Autodesk Inventor part; units mm, degrees
ref_plane "YZ Plane" through (0, 0, 0) normal (1, 0, 0) x (0, 1, 0)
ref_plane "XZ Plane" through (0, 0, 0) normal (0, 1, 0) x (-1, 0, 0)
ref_plane "XY Plane" through (0, 0, 0) normal (0, 0, 1) x (1, 0, 0)
sketch "Sketch1" plane through (0, 0, 0) normal (0, 0, 1) x (1, 0, 0)
  line L0 (-750, 48.2006) -> (750, 48.2006)
  line L1 (750, 48.2006) -> (750, 0)
  line L2 (750, 0) -> (-750, 0)
  line L3 (-750, 0) -> (-750, 48.2006)
  point P0 (0, 0)
  point P1 (0, 0)
  dimension "d0" = 1500
  dimension "d1" = 48.2006
extrude "Plate1" add sketch "Sketch1" along normal blind 3
sketch "Sketch2" plane through (750, 3, 0) normal (0, -1, 0) x (1, 0, 0)
  line L0 (-1500, 0) -> (0, 0)
  line L1 (0, 0) -> (0, 30)
  line L2 (0, 30) -> (-1500, 30)
  line L3 (-1500, 30) -> (-1500, 0)
edge flange "Flange1" height 30 angle 90 thickness 3 bend radius 3 thickness toward (0, -1, 0) relief tear relief width 3 relief depth 1.5 edges at (0, 0, 3) wall of the first edge with corners at (-750, 3, 0) (750, 3, 0) (750, 3, 30) (-750, 3, 30)
bend "Bend1"
corner "Corner1"
sketch "Sketch5" plane through (0, 0, 0) normal (0, 0, -1) x (-1, 0, 0)
  line L0 (750, 48.2006) -> (-750, 48.2006)
  line L1 (500, 48.2006) -> (500, 31)
  line L2 (500, 31) -> (503, 31)
  line L3 (503, 31) -> (503, 48.2006)
  line L4 (750, 0) -> (-750, 0)
  point P0 (0, 0)
  dimension "d18" = 3
  dimension "d19" = 247
  dimension "d20" = 31
extrude "Extrusion1" cut sketch "Sketch5" against normal through all
pattern_linear "Rectangular Pattern1" count 3 spacing 500 along (1, 0, 0) of "Extrusion1"
sketch "Sketch6" plane through (0, 0, 0) normal (0, 0, -1) x (-1, 0, 0)
  line L0 (-750, 48.2006) -> (-750, 6)
  circle A0 centre (-750, 48.2006) radius 15
  line L1 (-750, 48.2006) -> (-500, 48.2006)
  point P0 (0, 0)
  point P1 (-735, 48.2006)
  point P2 (-750, 33.2006)
  dimension "d24" = 30
extrude "Extrusion2" cut sketch "Sketch6" against normal through all contours L1 A0 L0 picked at (-740.1254, 47.088)
mirror "Mirror1" about plane through (0, 0, 0) normal (1, 0, 0) of "Extrusion2"
equation "\"d1\" = Стрингер_4"
equation "\"d18\" = Thickness"
equation "\"d2\" = Thickness"
equation "\"d3\" = BendReliefWidth"
equation "\"d4\" = BendReliefDepth"
equation "\"d5\" = MinimumRemnant"
equation "\"d6\" = TransitionRadius"
equation "\"d9\" = BendRadius"
equation "\"d10\" = CornerReliefSize"
equation "\"d11\" = GapSize"
equation "\"d12\" = JacobiRadiusSize"
equation "\"BendRadius\" = Thickness"
equation "\"BendReliefWidth\" = Thickness"
equation "\"BendReliefDepth\" = 0.5 * Thickness"
equation "\"CornerReliefSize\" = 4 * Thickness"
equation "\"MinimumRemnant\" = 2 * Thickness"
equation "\"TransitionRadius\" = BendRadius"
equation "\"JacobiRadiusSize\" = BendRadius"
equation "\"GapSize\" = Thickness"
properties part number "МОО 054 стрингер борт 41"
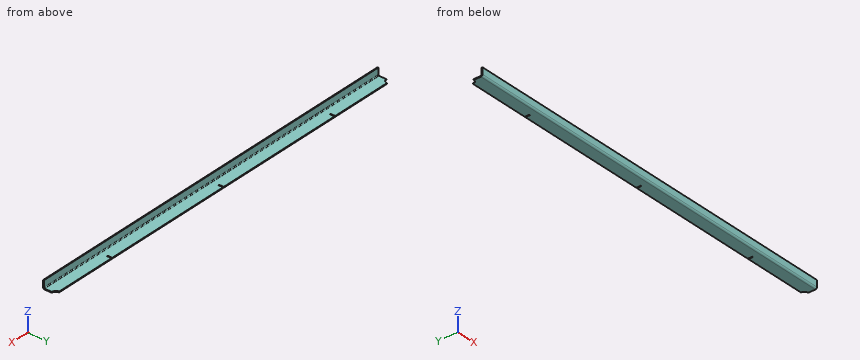
Input: part model. Units: mm. Frame: model coordinates. Give positions to 0.01 mm unless a question says otherwise; leave off trailing zeros. Order: outer loops, then holes, each group sorted by start corner. A loop starts at its lowest first (then second) coordinate and runs counter-clockwise, first axis right, second up. Notation, with made-up numbers: M -18.5,16.5 L 16.5,16.5 A29 ccw 16.5,41.5 Z; hole C -38.5,16.25 d7. An arc over 180 degrees is marked long. Return JSON: item names as keys, results as strings.
1) Line query: L1, parallel to Y at x = 185, z = 16.75; L2, parallel to Z at x = 522.5, y = 5. Output: solid intervals per line, ascending. Write a range as [from, to].
Taken from the geometry:
{"L1": "y = [0, 3]", "L2": "z = [0.08, 3.17]"}
2) Contact query for flat-ended pins moving along their axis: pin 1 (2.5 mm diameter, centred on y = 44, z = 1.5, fed in from -X); pin 2 (1.5 mm diameter, centred on x = -501, z = 1, fed in from +Y); pin 3 (1.5 mm diameter, centred on x = 46.5, z = 25, fed in from -Y); pin 4 (0.9 mm diameter, centred on y = 40.5, z = 2, fed in from -X). Output: stop coordinate, or through.
Taken from the geometry:
{"pin 1": "stops at x = -736.03", "pin 2": "stops at y = 31", "pin 3": "stops at y = 0", "pin 4": "stops at x = -737.41"}
3) Section query B-B on z = 12. Output: boundary loops of the cut face in (x, y).
Taken from the geometry:
{"outline": "M -750,0 L 750,0 L 750,3 L -750,3 Z"}
4) Section query A-A on x = 278. Output: boundary loops of the cut face in (y, z).
Taken from the geometry:
{"outline": "M 0,6 A6 ccw 6,0 L 48.2,0 L 48.2,3 L 6,3 A3 cw 3,6 L 3,30 L 0,30 Z"}
